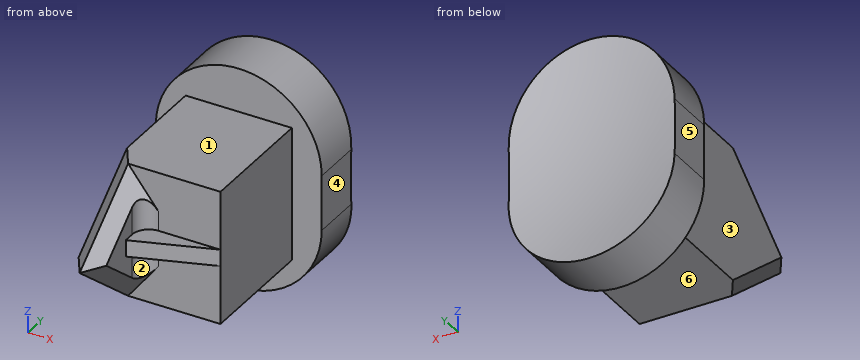
from build123d import *

# Parameters (mm, degrees)
SKETCH1_W           = 19.2
SKETCH1_H           = 24.2
BOSS_EXTRUDE1_DEPTH = 22.1
BOSS_EXTRUDE2_DEPTH = 10
BOSS_EXTRUDE3_DEPTH = 5
BOSS_EXTRUDE4_DEPTH = 1.5
CHAMFER1_SIZE       = 2.5
FILLET1_R           = 3


with BuildPart() as part:
    # Sketch1 → Boss-Extrude1 (new body)
    with BuildSketch(Plane(origin=(0, 0, 0), x_dir=(1, 0, 0), z_dir=(0, 1, 0))):
        Rectangle(SKETCH1_W, SKETCH1_H)
    extrude(amount=BOSS_EXTRUDE1_DEPTH)

    # Sketch2 → Boss-Extrude2 (add)
    with BuildSketch(Plane(origin=(0, 22.1, 0), x_dir=(1, 0, 0), z_dir=(0, 1, 0))):
        with BuildLine():
            Line((15, 5), (15, -5))
            ThreePointArc((15, -5), (0, -20), (-15, -5))
            Line((-15, -5), (-15, 5))
            ThreePointArc((-15, 5), (0, 20), (15, 5))
        make_face()
    extrude(amount=BOSS_EXTRUDE2_DEPTH)

    # Sketch4 → Boss-Extrude3 (add)
    with BuildSketch(Plane.ZY.offset(9.6)):
        Polygon((-12.1, 0), (0, -15), (12.1, 0), align=None)
    extrude(amount=-BOSS_EXTRUDE3_DEPTH)

    # Sketch6 → Boss-Extrude4 (add, symmetric)
    with BuildSketch(Plane.XY):
        Polygon((-4.6, -5), (9.6, 0), (-4.6, 0), align=None)
    extrude(amount=BOSS_EXTRUDE4_DEPTH, both=True)

    # Chamfer1
    chamfer1_edges = [part.edges().sort_by_distance(p)[0] for p in [
        (-9.6, -7.5, -6.05),
        (-4.6, -7.5, -6.05),
        (-9.6, -7.5, 6.05),
        (-4.6, -7.5, 6.05),
    ]]
    chamfer(chamfer1_edges, length=CHAMFER1_SIZE - 0.0001)  # a hair under: the kernel refuses the full size

    # Fillet1
    fillet1_edges = [part.edges().sort_by_distance(p)[0] for p in [
        (-4.6, 0, -5.194064205),
        (-4.6, 0, 5.194064205),
    ]]
    fillet(fillet1_edges, radius=FILLET1_R)

    # Sketch8 → Cut-Revolve3 (revolve, cut)
    with BuildSketch(Plane(origin=(0, 0, 0), x_dir=(0, 0, -1), z_dir=(1, 0, 0))):
        with BuildLine():
            Line((-90.14660282, 120), (90.14660282, 120))
            ThreePointArc((90.14660282, 120), (0, 29.85339718), (-90.14660282, 120))
        make_face()
    revolve(axis=Axis((0, 120, 90.14660282), (0, 0, -1)), mode=Mode.SUBTRACT)


solid = part.part
Design review of the part built by this model. Coordinates are the model's own, in mm. Face numbers are marked on the shaded views. A direction names the side the tool comes from. Round coordinates to 2 decimals unless told otherwise and drop trailing zeros. Write each loop counter-clockwise with the first axis right and the second up, starting at its lowest first coordinate (ties: lowest second). Pieces come first, ordered by that corner, then holes. Notation, with made-up numbers: (37, -31) -> (56, -31) arc R32 cw to (56, 7) -> close; hole circle Ø1 at (70, 62). An arc over 180 degrees is marked (long way). One line per item, written item: value. Start each with the question number.
Q1. Add section D-D (x = -3.5). Give the boundary of the cut face in (y, z).
Q2. Insertion check: P1, Ø12, axis at x = 9, y = 12.5, coming from the -Z side; P2, Ø8, axis at y = -4, z = -7.5, coming from the -X side; P3, Ø6, axis at x = -3, z = 10.5, coming from the -Y side. Each pin has a flat end and moves straight along its axis. Give the tip position at first contact, or say it passes through.
Q3. To check wall thickness, follow probe 1 along X at (y, z) = (21, 6); probe 2 along Y at (x, z) = (-11, -9.5); probe 3 along Z at (x, y) = (0, 20). State the ranges of each line that lie inside material, in increasing order.
Q4. Add section C-C (y = 12). Give the boundary of the cut face in (x, z).
Q5. Tool access review of the marked faces 1, 2 and 3: name each direction out of +Z, -Z, +X, -X, +Y, -Y from which nothing blocks a thin tool from reaching the whole face with its end or side.
Q6. The part is to be moulded in two halves that separate along X. For the marked faces 4, 5 and 6, say which applies: pulls with the +X half, pulls with the -X half, needs draft (parallel to the pull), parting line crosses it, or undercut.
Q7. Add section A-A (x = 0). Give the boundary of the cut face in (y, z), then the cut area to 3 significant figures.
Response:
1. outline: (-4.61, -1.5) -> (-0.68, -1.5) -> (-0.68, -6.93) -> (0, -7.47) -> (0, -12.1) -> (22.1, -12.1) -> (22.1, -19.59) -> (32.08, -19.59) arc R90.08 cw to (32.08, 19.59) -> (22.1, 19.59) -> (22.1, 12.1) -> (0, 12.1) -> (0, 7.47) -> (-0.68, 6.93) -> (-0.68, 1.5) -> (-4.61, 1.5) -> close
2. P1: stops at z = -12.1
2. P2: stops at x = -9.6
2. P3: stops at y = -1.51
3. probe 1: x = -9.6 to 9.6
3. probe 2: y = 22.1 to 31.03
3. probe 3: z = -12.1 to 12.1
4. outline: (-9.6, -12.1) -> (9.6, -12.1) -> (9.6, 12.1) -> (-9.6, 12.1) -> close
5. face 1: +Z, +X, -X, -Y
5. face 2: -Z, +X, -Y
5. face 3: +Z, -Z, -X, -Y
6. face 4: pulls with the +X half
6. face 5: pulls with the -X half
6. face 6: needs draft
7. outline: (-3.38, -1.5) -> (0, -1.5) -> (0, -12.1) -> (22.1, -12.1) -> (22.1, -20) -> (32.1, -20) arc R90.15 cw to (32.1, 20) -> (22.1, 20) -> (22.1, 12.1) -> (0, 12.1) -> (0, 1.5) -> (-3.38, 1.5) -> close
7. area: 885 mm^2
